```python
from build123d import *

# Parameters (mm, degrees)
SKETCH1_W              = 254
SKETCH1_H              = 88.9
BOSS_EXTRUDE1_DEPTH    = 6
F_10_CLEARANCE_HOLE1_D = 6.0452
M22_CLEARANCE_HOLE1_D  = 26


with BuildPart() as part:
    # Sketch1 → Boss-Extrude1 (new body)
    with BuildSketch(Plane.YZ):
        Rectangle(SKETCH1_W, SKETCH1_H)
    extrude(amount=-BOSS_EXTRUDE1_DEPTH)

    # #10 Clearance Hole1 (through all)
    with Locations(Plane.YZ):
        with Locations((118.2625, 38.1), (-118.2625, 38.1), (-118.2625, -38.1), (118.2625, -38.1)):
            Hole(F_10_CLEARANCE_HOLE1_D / 2)

    # M22 Clearance Hole1 (through all)
    with Locations(Plane.YZ):
        with Locations((87, 0), (29, 0), (-29, 0), (-87, 0)):
            Hole(M22_CLEARANCE_HOLE1_D / 2)


solid = part.part
```
Can you work these out from the model? Positions are in its coordinate system, mm. Give positions to 0.01 mm unless a question says otherwise; leave off trailing zeros. Loops run counter-clockwise (first coordinate to the right, second up) from the corner with the lowest first, then second, coordinate; pieces in that order, holes last. Notation, with made-up numbers: M -12.75,52 L 0.25,52 A10 ccw 0.25,68 Z; hole C -33,21 d8. An arc over 180 degrees is marked long. Use one line per item in the form item = value. Start each with the question number.
(1) I want a section at D-D, the plane z = 0. Write out the boundary of the cut face in (x, y), and give its area (3 significant figures).
(2) Thinking about a two-plate mould opening in Y: for faces 1 (the cylindrical face through (-3.04, -117.61, 35.15)), 2 (the flat face through (-3, 127, -1)), 3 (the flat face through (-3, -2, -44.45)), which applies, released by +Y, released by -Y, zero draft, split by the parting line, or undercut?
(3) I want a section at A-A, the plane y = -29. Write out the boundary of the cut face in (x, z), and give its area (3 significant figures).
(4) I want a section at B-B, the plane z = -38.1. Write out the boundary of the cut face in (x, y).
(5) I want a section at C-C, the plane x = -4.9. State how many separate pieces and enclosed holes the cut face has, and give its area (3 significant figures).
(6) Please list where these lines run through material, in increasing order: line 1 (Y direction, x = -1.45, z = -38.5); line 2 (Z direction, x = -3.65, y = 29); line 3 (Y direction, x = -2.4, z = 4).
Worked out:
q1.outline = M -6,-127 L 0,-127 L 0,-100 L -6,-100 Z; M -6,-74 L 0,-74 L 0,-42 L -6,-42 Z; M -6,-16 L 0,-16 L 0,16 L -6,16 Z; M -6,42 L 0,42 L 0,74 L -6,74 Z; M -6,100 L 0,100 L 0,127 L -6,127 Z
q1.area = 900 mm²
q2.face_1 = undercut
q2.face_2 = released by +Y
q2.face_3 = zero draft
q3.outline = M -6,-44.45 L 0,-44.45 L 0,-13 L -6,-13 Z; M -6,13 L 0,13 L 0,44.45 L -6,44.45 Z
q3.area = 377 mm²
q4.outline = M -6,-127 L 0,-127 L 0,-121.29 L -6,-121.29 Z; M -6,-115.24 L 0,-115.24 L 0,115.24 L -6,115.24 Z; M -6,121.29 L 0,121.29 L 0,127 L -6,127 Z
q5.separate_pieces = 1
q5.enclosed_holes = 8
q5.area = 20,300 mm²
q6.line_1 = -127 to -121.26, -115.27 to 115.27, 121.26 to 127
q6.line_2 = -44.45 to -13, 13 to 44.45
q6.line_3 = -127 to -99.37, -74.63 to -41.37, -16.63 to 16.63, 41.37 to 74.63, 99.37 to 127
